from build123d import *

# Parameters (mm, degrees)
BOSS_EXTRUDE1_DEPTH      = 6.35
FILLET1_R                = 12.7
CUT_EXTRUDE2_DEPTH       = 3.175
BOSS_EXTRUDE2_DEPTH      = 3.175
BOSS_EXTRUDE2_DEPTH_BACK = 36.135303
SKETCH4_R                = 9.525
SKETCH4_R_2              = 6.35
SKETCH5_R                = 9.525
SKETCH5_R_2              = 6.35
BOSS_EXTRUDE3_DEPTH      = 25.4
CHAMFER2_SIZE            = 1
CHAMFER4_SIZE            = 1


with BuildPart() as part:
    # Sketch1 → Boss-Extrude1 (new, symmetric)
    with BuildSketch(Plane.YZ):
        Polygon((-25.4, 10.735303163), (0, 25.4), (25.4, 25.4), (25.4, -25.4), (-25.4, -25.4), align=None)
    extrude(amount=BOSS_EXTRUDE1_DEPTH, both=True)

    # Fillet1
    fillet1_edges = [part.edges().sort_by_distance(p)[0] for p in [
        (0, 25.4, -25.4),
    ]]
    fillet(fillet1_edges, radius=FILLET1_R)

    # Sketch3 → Cut-Extrude2 (cut)
    with BuildSketch(Plane.YZ.offset(6.35)):
        with BuildLine():
            Line((-22.225, -22.225), (12.7, -22.225))
            ThreePointArc((12.7, -22.225), (19.435192091, -19.435192091), (22.225, -12.7))
            Line((22.225, -12.7), (22.225, 22.225))
            Line((22.225, 22.225), (0.850738686, 22.225))
            Line((0.850738686, 22.225), (-22.225, 8.902216058))
            Line((-22.225, 8.902216058), (-22.225, -22.225))
        make_face()
    extrude(amount=-CUT_EXTRUDE2_DEPTH, mode=Mode.SUBTRACT)

    # Sketch4 → Boss-Extrude2 (add, two sides: drawn at the far end of the back side and taken through both)
    with BuildSketch(Plane(origin=(0, 0, -25.4), x_dir=(1, 0, 0), z_dir=(0, 0, -1)).offset(-BOSS_EXTRUDE2_DEPTH_BACK)):
        with Locations(Location((0, 33.02, 0), (0, 0, 233.130102354))):
            Circle(SKETCH4_R)
        with Locations(Location((0, 33.02, 0), (0, 0, 270))):
            Circle(SKETCH4_R_2, mode=Mode.SUBTRACT)
    extrude(amount=BOSS_EXTRUDE2_DEPTH + BOSS_EXTRUDE2_DEPTH_BACK)

    # Sketch5 → Boss-Extrude3 (add)
    with BuildSketch(Plane(origin=(0, 25.4, 0), x_dir=(-1, 0, 0), z_dir=(0, 1, 0))):
        with Locations((0, 33.02)):
            Circle(SKETCH5_R)
        with Locations(Location((0, 33.02, 0), (0, 0, 90))):
            Circle(SKETCH5_R_2, mode=Mode.SUBTRACT)
    extrude(amount=-BOSS_EXTRUDE3_DEPTH)

    # Chamfer2
    # the kernel refuses this chamfer: 1 mm, written as the material it takes off along each edge
    with BuildSketch(Plane(origin=(0, -33.02, 10.735303), x_dir=(0.3638595085405839, 0.931453841070294, 0), z_dir=(-0.931453841070294, 0.3638595085405839, 0))) as chamfer2_piece_1_section:
        Polygon((9.525, CHAMFER2_SIZE), (9.525 - CHAMFER2_SIZE, 0), (9.525, 0), align=None)
    chamfer2_piece_1 = revolve(axis=Axis((0, -33.02, 10.735303), (0, 0, -1)), revolution_arc=317.325176487, mode=Mode.PRIVATE)
    chamfer2_piece_1 = split(chamfer2_piece_1, bisect_by=Plane(origin=(5.777045626, -25.4, 10.24862198), z_dir=(0, -1, 0)), keep=Keep.TOP, mode=Mode.PRIVATE)
    add(chamfer2_piece_1, mode=Mode.SUBTRACT)
    with BuildSketch(Plane(origin=(0, -33.02, -28.575), x_dir=(-0.6000000000021781, 0.7999999999983665, 0), z_dir=(-0.7999999999983665, -0.6000000000021781, 0))) as chamfer2_piece_2:
        Polygon((9.525, -CHAMFER2_SIZE), (9.525 - CHAMFER2_SIZE, 0), (9.525, 0), align=None)
    revolve(axis=Axis((0, -33.02, -28.575), (0, 0, -1)), mode=Mode.SUBTRACT)
    with BuildSketch(Plane(origin=(0, 25.4, 33.02), x_dir=(-0.3638595085405501, 0, -0.9314538410703074), z_dir=(0.9314538410703074, 0, -0.3638595085405501))) as chamfer2_piece_3_section:
        Polygon((9.525, -CHAMFER2_SIZE), (9.525 - CHAMFER2_SIZE, 0), (9.525, 0), align=None)
    chamfer2_piece_3 = revolve(axis=Axis((0, 25.4, 33.02), (0, 1, 0)), revolution_arc=317.325176487, mode=Mode.PRIVATE)
    chamfer2_piece_3 = split(chamfer2_piece_3, bisect_by=Plane(origin=(0, 24.920234358, 25.4), z_dir=(0, 0, 1)), keep=Keep.TOP, mode=Mode.PRIVATE)
    add(chamfer2_piece_3, mode=Mode.SUBTRACT)
    with BuildSketch(Plane(origin=(0, 0, 33.02), x_dir=(-0.3638595085405531, 0, -0.9314538410703063), z_dir=(0.9314538410703063, 0, -0.3638595085405531))) as chamfer2_piece_4_section:
        Polygon((9.525, CHAMFER2_SIZE), (9.525 - CHAMFER2_SIZE, 0), (9.525, 0), align=None)
    chamfer2_piece_4 = revolve(axis=Axis((0, 0, 33.02), (0, 1, 0)), revolution_arc=317.325176487, mode=Mode.PRIVATE)
    chamfer2_piece_4 = split(chamfer2_piece_4, bisect_by=Plane(origin=(-5.452412952, 0.490850729, 25.4), z_dir=(0, 0, 1)), keep=Keep.TOP, mode=Mode.PRIVATE)
    add(chamfer2_piece_4, mode=Mode.SUBTRACT)

    # Sweep3: sweep along a path in Sketch6
    with BuildLine(Plane.YZ) as sweep3_path:
        Line((0, 33.02), (-20.32, 33.02))
        ThreePointArc((-20.32, 33.02), (-29.300256121, 29.300256121), (-33.02, 20.32))
        Line((-33.02, 20.32), (-33.02, 10.735303163))
    # Sketch7 → Sweep3 (sweep)
    with BuildSketch(Plane.XZ):
        with BuildLine():
            Line((-8.525, 33.02), (-6.35, 33.02))
            ThreePointArc((-6.35, 33.02), (0, 26.67), (6.35, 33.02))
            Line((6.35, 33.02), (8.525, 33.02))
            ThreePointArc((8.525, 33.02), (0, 24.495), (-8.525, 33.02))
        make_face()
    sweep(path=sweep3_path.line)

    # Chamfer4
    chamfer4_edges = [part.edges().sort_by_distance(p)[0] for p in [
        (3.175, -22.225, -6.661391971),
        (3.175, -10.687130657, 15.563608029),
        (3.175, 11.537869343, 22.225),
        (3.175, 22.225, 4.7625),
        (3.175, 19.435192091, -19.435192091),
        (3.175, -4.7625, -22.225),
    ]]
    chamfer(chamfer4_edges, length=CHAMFER4_SIZE)


solid = part.part
Geometry: final body of the model. Coordinates: model frame, mm. A direction names the side the tool comes from. Coordinates: 2 decimals unless noted, no trailing zeros. Loops run counter-clockwise (first coordinate to the right, second up) from the corner with the lowest first, then second, coordinate; pieces in that order, holes last. Notation, with made-up numbers: (75.25, -21.75) - (110.25, -21.75) arc R22 ccw to (110.25, 6.25) - close; hole circle Ø10 at (21.25, 35.5). An arc over 180 degrees is marked (long way). Put each result on its own line as item: value. Start each with the question number.
Q1. Cut plane A-A, the plane x = 0. Give the number of separate pieces and of enclosed holes in the cut face, and give its area (3 significant figures).
Q2. Line query: line 1 (Z direction, x = 0, y = 12) (3 decimals); line 2 (Z direction, x = 4.5, y = -13) (3 decimals); line 3 (Y direction, x = -0.25, z = 4.5). Output: solid intervals per line, ascending.
Q3. Pull-direction query (Z, two-part tool) for faces 1 (the flat face through (0.089, -12.878, 17.965)), 2 (the flat face through (-7, -10, 33.02)), 3 (the flat face through (-6.35, 0, 0)); classes: released by +Z, released by -Z, zero draft, split by the parting line, or undercut.
Q4. Pin query (flat end, axial travel): pin 1 Ø8 at (y, z) = (-13, 34.5) entering from +X (3 decimals); pin 2 Ø1.3 at (x, z) = (-5, -8.5) entering from -Y; pin 3 Ø7.5 at (x, y) = (0, -33.02) entering from +Z; pin 4 Ø1.1 at (x, y) = (7.5, -13) entering from +Z. Return the tip coordinate at first contact, or that it passes through.
Q5. Cut plane D-D, the plane y = 3.5. Return loops of the section in (x, z) (3 decimals), and give its area (3 significant figures).
Q6. Cut plane C-C, the plane z = -11. Return loops of the section in (x, y) (3 decimals).
Q7. Set-up query: faces 4 (the flat face through (7, -10, 33.02)), 5 (the flat face through (5, -5, -22.225)), 6 (the cylindrical face through (0.09, 21.58, -21.78)). Return all of +Z, -Z, +X, -X, +Y, -Y with unobstructed straight access to the full face (end or side cutting, diameter ignored); none if empty.
Q8. Cut plane B-B, the plane y = -8. Return loops of the section in (x, z) (3 decimals), and give its area (3 significant figures).
Filled sheet:
1. separate pieces: 3
1. enclosed holes: 1
1. area: 2,730 mm²
2. line 1: -25.4 to 26.67, 39.37 to 42.545
2. line 2: -25.4 to -22.225, 14.228 to 17.894, 25.779 to 28.54
2. line 3: -42.54 to -39.37, -26.67 to 25.4
3. face 1: undercut
3. face 2: released by +Z
3. face 3: zero draft
4. pin 1: x = 8.525
4. pin 2: y = -41.49
4. pin 3: through
4. pin 4: z = 33.02
5. outline: (-6.35, -25.4) - (6.35, -25.4) - (6.35, -22.225) - (4.175, -22.225) - (3.175, -21.225) - (3.175, 21.225) - (4.175, 22.225) - (6.35, 22.225) - (6.35, 25.4) - (5.715, 25.4) arc R9.525 ccw (long way) to (-5.715, 25.4) - (-6.35, 25.4) - close; hole circle Ø12.7 at (0, 33.02)
5. area: 649 mm²
6. outline: (-6.35, -25.4) - (-5.715, -25.4) arc R9.525 ccw (long way) to (5.715, -25.4) - (6.35, -25.4) - (6.35, -22.225) - (4.175, -22.225) - (3.175, -21.225) - (3.175, 21.225) - (4.175, 22.225) - (6.35, 22.225) - (6.35, 25.4) - (-6.35, 25.4) - close; hole circle Ø12.7 at (0, -33.02)
7. face 4: +Z, +X, -X, -Y
7. face 5: +X
7. face 6: -Z, +X, -X, +Y
8. outline: (-8.525, 33.02) arc R8.525 ccw to (8.525, 33.02) - (6.35, 33.02) arc R6.35 cw to (-6.35, 33.02) - close; (-6.35, -25.4) - (6.35, -25.4) - (6.35, -22.225) - (4.175, -22.225) - (3.175, -21.225) - (3.175, 15.96) - (4.175, 17.115) - (6.35, 17.115) - (6.35, 20.781) - (-6.35, 20.781) - close
8. area: 513 mm²
